```python
from build123d import *

# Parameters (mm, degrees)
F1_DEPTH       = 76.2
F3_DEPTH       = 27.94
F5_D           = 15.24
F5_CBORE_D     = 40.64
F5_CBORE_DEPTH = 10.16
F6_W           = 10.16
F6_H           = 10.16
F7_DEPTH       = 76.2
F8_R           = 10.16
F9_DEPTH       = 76.201
F10_R          = 10.16


with BuildPart() as f1:
    # F0 (on Front) → F1 (new body)
    with BuildSketch(Plane.XZ):
        Polygon((-28.956, 28.956), (0, 0), (118.364, 0), (118.364, 35.56), (42.164, 35.56), (6.604, 71.12), (-28.956, 71.12), align=None)
    extrude(amount=F1_DEPTH)

    # F2 (on face) → F3 (cut)
    with BuildSketch(Plane.XY.offset(71.12)):
        with BuildLine():
            ThreePointArc((-11.176, -7.62), (-16.564154, -9.851846), (-18.796, -15.24))
            Line((-18.796, -15.24), (-18.796, -60.96))
            ThreePointArc((-18.796, -60.96), (-16.564154, -66.348154), (-11.176, -68.58))
            ThreePointArc((-11.176, -68.58), (-5.787846, -66.348154), (-3.556, -60.96))
            Line((-3.556, -60.96), (-3.556, -15.24))
            ThreePointArc((-3.556, -15.24), (-5.787846, -9.851846), (-11.176, -7.62))
        make_face()
    extrude(amount=-F3_DEPTH, mode=Mode.SUBTRACT)

    # F5 (through all)
    with Locations(Plane.XY.offset(35.56)):
        with Locations((80.264, -38.1)):
            CounterBoreHole(F5_D / 2, F5_CBORE_D / 2, F5_CBORE_DEPTH)

    # F6 (on face) → F7 (cut)
    with BuildSketch(Plane.YZ.offset(118.364)):
        with Locations((-38.1, 30.48)):
            Rectangle(F6_W, F6_H)
    extrude(amount=-F7_DEPTH, mode=Mode.SUBTRACT)

    # F8 (on face) → F9 (cut, through all)
    with BuildSketch(Plane(origin=(0, 0, 0), x_dir=(-1, 0, 0), z_dir=(0, 1, 0))):
        with Locations((-24.384, 20.32)):
            Circle(F8_R)
    extrude(amount=-F9_DEPTH, mode=Mode.SUBTRACT)

    # F10
    f10_edges = [f1.edges().sort_by_distance(p)[0] for p in [
        (118.364, -76.2, 17.78),
        (118.364, 0, 17.78),
    ]]
    fillet(f10_edges, radius=F10_R)


solid = f1.part
```
Geometry check sheet. Reference: the model listing, model coordinates, mm. A direction names the side the tool comes from. Coordinates: 2 decimals unless noted, no trailing zeros. Order: outer loops, then holes, each group sorted by start corner. A loop starts at its lowest first (then second) coordinate and runs counter-clockwise, first axis right, second up. Notation, with made-up numbers: M 84,-7.75 L 139,-7.75 A26 ccw 139,29.25 Z; hole C -32,24 d6. An arc over 180 degrees is marked long. One line per question, with ' | ' between items. Start each with the question number.
Item 1: Cross-section at C-C on z = 63.5. Enter the section's corners in (x, y), then the cut area to 3 significant figures.
Item 2: Gauge pin test, flat ends, axial feed: pin 1 (16.5 mm diameter, centred on x = 69.5, y = -53, fed in from +Z); pin 2 (17.5 mm diameter, centred on x = 80.264, y = -38.1, fed in from -Z); pin 3 (2 mm diameter, centred on x = 87.5, y = -42, fed in from +Z); pin 4 (22.5 mm diameter, centred on y = -33.5, z = 57.5, fed in from +X). Record the tip position at first contact, or that the pin passes through.
Item 3: Cross-section at D-D on x = 81. Enter the section's corners in (y, z).
Item 4: Draft check along Z on faces 5 (the cylindrical face through (26.586, -37.567, 10.402)), 6 (the flat face through (109, -33.02, 30)), 7 (the flat face through (24.633, -37.567, 53.091)). Enter one of: pulls with the +Z half, pulls with the -Z half, needs draft (parallel to the pull), parting line crosses it, or undercut.
Item 5: Material ranges on L1, parallel to Y at x = 81, z = 19; L2, parallel to Z at x = 54.5, y = -13; L3, parallel to Y at x = -16, z = 64.5, recorded low to high. Write a range as [from, to].
Item 6: Cross-section at B-B on y = -38.1. Enter the section's corners in (x, z).
Item 7: Set-up check for faces 1 (the flat face through (-3, -38, 71.12)), 2 (the flat face through (81, -63, 35.56)), 3 (the flat face through (42.164, -38, 31)), 4 (the flat face through (72, -38, 25.4)): record each of +Z, -Z, +X, -X, +Y, -Y from which the full face is reachable in a straight line by a thin tool's end or side.
Item 8: Cross-section at A-A on z = 20.32. Enter the section's corners in (x, y).
Findings:
1) outline: M -28.96,-76.2 L 14.22,-76.2 L 14.22,0 L -28.96,0 Z; hole M -18.8,-60.96 A7.62 ccw -11.18,-68.58 A7.62 ccw -3.56,-60.96 L -3.56,-15.24 A7.62 ccw -11.18,-7.62 A7.62 ccw -18.8,-15.24 Z | area: 2,410 mm²
2) pin 1: stops at z = 35.56 | pin 2: stops at z = 0 | pin 3: stops at z = 25.4 | pin 4: stops at x = 31.47
3) outline: M -76.2,0 L -45.68,0 L -45.68,25.4 L -58.41,25.4 L -58.41,35.56 L -76.2,35.56 Z; M -30.52,0 L 0,0 L 0,35.56 L -17.79,35.56 L -17.79,25.4 L -30.52,25.4 Z
4) face 5: undercut | face 6: needs draft | face 7: pulls with the +Z half
5) L1: y = [-76.2, -45.68], [-30.52, 0] | L2: z = [0, 35.56] | L3: y = [-76.2, -66.86], [-9.34, 0]
6) outline: M -28.96,28.96 L 0,0 L 72.64,0 L 72.64,25.4 L 42.16,25.4 L 42.16,35.56 L 6.6,71.12 L -3.56,71.12 L -3.56,43.18 L -18.8,43.18 L -18.8,71.12 L -28.96,71.12 Z; M 87.88,0 L 118.36,0 L 118.36,25.4 L 87.88,25.4 Z; hole C 24.38,20.32 d20.32
7) face 1: +Z, +X, -X, +Y, -Y | face 2: +Z, +X, +Y, -Y | face 3: +Z, +X | face 4: +Z
8) outline: M -20.32,-76.2 L 14.22,-76.2 L 14.22,0 L -20.32,0 Z; M 34.54,-76.2 L 108.2,-76.2 A10.16 ccw 118.36,-66.04 L 118.36,-10.16 A10.16 ccw 108.2,0 L 34.54,0 Z; hole C 80.26,-38.1 d15.24
